```python
from build123d import *

# Parameters (mm, degrees)
F1_DEPTH = 6.858
F2_R     = 1.75
F3_DEPTH = 6.859
F4_R     = 1
F5_R     = 2
F6_R     = 0.5
F7_R     = 1
F8_R     = 1.6
F9_R     = 1.6
F10_R    = 1.6


with BuildPart() as f1:
    # F0 (on Top) → F1 (new body)
    with BuildSketch(Plane.XY):
        with BuildLine():
            ThreePointArc((0, 2), (0.585786, 0.585786), (2, 0))
            Line((2, 0), (2.5, 0))
            ThreePointArc((2.5, 0), (2.84202, 0.060307), (3.142788, 0.233956))
            Line((3.142788, 0.233956), (12.614652, 8.181793))
            Line((12.614652, 8.181793), (18.796832, 8.181793))
            ThreePointArc((18.796832, 8.181793), (20.21605, 7.320591), (20.107475, 5.664071))
            Line((20.107475, 5.664071), (17.191762, 1.5))
            Line((17.191762, 1.5), (15.69747, 1.630734))
            Line((15.69747, 1.630734), (16.638974, 0))
            Line((16.638974, 0), (24.396832, 0))
            Line((24.396832, 0), (24.396832, 6.581793))
            Line((24.396832, 6.581793), (30.096832, 9.87269))
            Line((30.096832, 9.87269), (35.796832, 6.581793))
            Line((35.796832, 6.581793), (35.796832, 0))
            Line((35.796832, 0), (39.796832, 0))
            Line((39.796832, 0), (39.796832, 4.618802))
            Line((39.796832, 4.618802), (43.796832, 6.928203))
            Line((43.796832, 6.928203), (47.796832, 4.618802))
            Line((47.796832, 4.618802), (47.796832, 0))
            Line((47.796832, 0), (51.796832, 0))
            Line((51.796832, 0), (51.796832, 19.87269))
            ThreePointArc((51.796832, 19.87269), (50.796832, 21.60474), (48.796832, 21.60474))
            Line((48.796832, 21.60474), (34.286578, 13.227241))
            Line((34.286578, 13.227241), (31.436578, 14.87269))
            Line((31.436578, 14.87269), (30.096832, 14.87269))
            Line((30.096832, 14.87269), (12.66367, 14.87269))
            Line((12.66367, 14.87269), (6.374878, 9.595767))
            ThreePointArc((6.374878, 9.595767), (3.909422, 9.811466), (4.125122, 12.276923))
            Line((4.125122, 12.276923), (11.389774, 18.37269))
            Line((11.389774, 18.37269), (32.3744, 18.37269))
            Line((32.3744, 18.37269), (34.286578, 17.268693))
            Line((34.286578, 17.268693), (42.260934, 21.87269))
            Line((42.260934, 21.87269), (0, 21.87269))
            Line((0, 21.87269), (0, 2))
        make_face()
        Polygon((49.796832, 7.505553), (39.086578, 13.689122), (49.796832, 19.87269), align=None, mode=Mode.SUBTRACT)
    extrude(amount=F1_DEPTH)

    # F2 (on face) → F3 (cut, through all)
    with BuildSketch(Plane.XY.offset(6.858)):
        with Locations((30.096832, 8.12269)):
            Circle(F2_R)
        with Locations((34.281288, 5.706793)):
            Circle(F2_R)
        with Locations((25.912377, 5.706793)):
            Circle(F2_R)
        with BuildLine():
            ThreePointArc((45.540307, 5.329188), (45.5452, 5.253766), (45.546832, 5.178203))
            ThreePointArc((45.546832, 5.178203), (45.273182, 4.23858), (44.537813, 3.592818))
            ThreePointArc((44.537813, 3.592818), (46.35685, 1.995434), (48.031288, 3.743802))
            ThreePointArc((48.031288, 3.743802), (47.220911, 5.220152), (45.540307, 5.329188))
        make_face()
        with BuildLine():
            ThreePointArc((44.537813, 3.592818), (44.765743, 4.618802), (45.540307, 5.329188))
            ThreePointArc((45.540307, 5.329188), (43.796832, 6.928203), (42.053358, 5.329188))
            ThreePointArc((42.053358, 5.329188), (42.788726, 4.683425), (43.062377, 3.743802))
            ThreePointArc((43.062377, 3.743802), (43.060745, 3.668239), (43.055851, 3.592818))
            ThreePointArc((43.055851, 3.592818), (43.796832, 3.428203), (44.537813, 3.592818))
        make_face()
        with BuildLine():
            ThreePointArc((43.055851, 3.592818), (42.281288, 4.303203), (42.053358, 5.329188))
            ThreePointArc((42.053358, 5.329188), (39.796832, 2.868802), (43.055851, 3.592818))
        make_face()
    extrude(amount=-F3_DEPTH, mode=Mode.SUBTRACT)

    # F4
    f4_edges = [f1.edges().sort_by_distance(p)[0] for p in [
        (24.396832, 0, 3.429),
        (35.796832, 0, 3.429),
        (39.796832, 0, 3.429),
        (47.796832, 0, 3.429),
    ]]
    fillet(f4_edges, radius=F4_R)

    # F5
    f5_edges = [f1.edges().sort_by_distance(p)[0] for p in [
        (51.796832, 0, 3.429),
        (0, 21.87269, 3.429),
    ]]
    fillet(f5_edges, radius=F5_R)

    # F6
    f6_edges = [f1.edges().sort_by_distance(p)[0] for p in [
        (42.260934, 21.87269, 3.429),
    ]]
    fillet(f6_edges, radius=F6_R)

    # F7
    f7_edges = [f1.edges().sort_by_distance(p)[0] for p in [
        (12.66367, 14.87269, 3.429),
        (31.436578, 14.87269, 3.429),
    ]]
    fillet(f7_edges, radius=F7_R)

    # F8
    f8_edges = [f1.edges().sort_by_distance(p)[0] for p in [
        (39.086578, 13.689122, 3.429),
        (49.796832, 19.87269, 3.429),
        (49.796832, 7.505553, 3.429),
    ]]
    fillet(f8_edges, radius=F8_R)

    # F9
    f9_edges = [f1.edges().sort_by_distance(p)[0] for p in [
        (17.191762, 1.5, 3.429),
    ]]
    fillet(f9_edges, radius=F9_R)

    # F10
    f10_edges = [f1.edges().sort_by_distance(p)[0] for p in [
        (34.286578, 13.227241, 3.429),
        (32.3744, 18.37269, 3.429),
        (11.389774, 18.37269, 3.429),
        (12.614652, 8.181793, 3.429),
    ]]
    fillet(f10_edges, radius=F10_R)


solid = f1.part
```
Source: CAD feature listing. Evaluate the final solid. Frame: model axes, mm. A direction names the side the tool comes from. Round coordinates to 2 decimals unless told otherwise and drop trailing zeros. Loops run counter-clockwise (first coordinate to the right, second up) from the corner with the lowest first, then second, coordinate; pieces in that order, holes last.
1. Ray query, L1, parallel to X at y = 17, z = 1.5; L2, parallel to X at y = 15, z = 1.25; L3, parallel to X at y = 6, z = 2. Return the intervals inside material, ascending.
2. Section query A-A on x = 5.25. Output: boundary loops of the cut face in (y, z), and give its area (3 significant figures).
3. Mould query, pull axis Y, two halves, no side actions, for faces 1 (the flat face through (32.928, 8.238, 3.381)), 2 (the flat face through (21, 21.873, 3)), 3 (the flat face through (44.483, 10.573, 3.381)). Classes: released by +Y, released by -Y, zero draft, split by the parting line, or undercut.
4. Access query for faces 4 (the flat face through (45.79, 5.777, 3.381)), 5 (the flat face through (51.797, 11, 3)), 6 (the flat face through (37.42, 19.08, 3.38)). Directions: +Z, -Z, +X, -X, +Y, -Y. A direction counts if a zero-diameter tool reaches every point of the face in a straight line with its end or side. Return the directions, or none.
Answers below:
1. L1: x = 0 to 9.75, 40.82 to 44.82, 49.8 to 51.8
1. L2: x = 0 to 7.37, 37.36 to 41.37, 49.8 to 51.8
1. L3: x = 0 to 10.01, 20.29 to 24.19, 36.01 to 42.19, 45.4 to 51.8
2. outline: (2, 0) - (9.19, 0) - (9.19, 6.86) - (2, 6.86) - close; (13.22, 0) - (21.87, 0) - (21.87, 6.86) - (13.22, 6.86) - close
2. area: 109 mm2
3. face 1: released by -Y
3. face 2: released by +Y
3. face 3: undercut
4. face 4: +Z, -Z, -Y
4. face 5: +Z, -Z, +X, +Y, -Y
4. face 6: +Z, -Z
